Work out the finished part from the listing and answer in its coordinate system (mm). A direction names the side the tool comes from. Give positions to 0.01 mm unless a question says otherwise; leave off trailing zeros. Write each loop counter-clockwise with the first axis right and the second up, starting at its lowest first coordinate (ties: lowest second). Pieces come first, ordered by that corner, then holes. Notation, with made-up numbers: (38, 78) - (64, 78) arc R22 cw to (64, 108) - close; hole circle Ø6 at (-35.75, 40.5). An arc over 180 degrees is marked (long way). Write item = value, one per line.
from build123d import *

# Parameters (mm, degrees)
SKETCH1_W               = 48
SKETCH1_H               = 6
BOSS_EXTRUDE1_DEPTH     = 205
FILLET1_R               = 25
SKETCH2_R               = 2.55
CUT_EXTRUDE1_DEPTH      = 207.487287744
LPATTERN1_COUNT         = 10
LPATTERN1_PITCH         = 10
CUT_EXTRUDE2_DEPTH      = 207.421898063
CUT_EXTRUDE2_DEPTH_BACK = 207.421898063
SKETCH12_W              = 15
SKETCH12_H              = 55
FILLET2_R               = 5


with BuildPart() as part:
    # Sketch1 → Boss-Extrude1 (new body)
    with BuildSketch(Plane(origin=(0, 0, 0), x_dir=(1, 0, 0), z_dir=(0, 1, 0))):
        Rectangle(SKETCH1_W, SKETCH1_H)
    extrude(amount=BOSS_EXTRUDE1_DEPTH)

    # Fillet1
    # the kernel refuses this fillet: 25 mm, written as the material it takes off along each edge
    with BuildSketch(Plane(origin=(-24, 0, 65.5), x_dir=(0, 1, 0), z_dir=(0, 0, -1)), Plane(origin=(24, 0, -65.5), x_dir=(0, 1, 0), z_dir=(0, 0, 1))) as fillet1_piece_1:
        with BuildLine():
            CenterArc((FILLET1_R, FILLET1_R), FILLET1_R, 180, 90)
            Line((0, FILLET1_R), (0, 0))
            Line((0, 0), (FILLET1_R, 0))
        make_face()
    extrude(amount=131, mode=Mode.SUBTRACT)

    # Sketch2 → Cut-Extrude1 (cut, through all)
    with BuildSketch(Plane.XY.offset(3)):
        with Locations((0, 12.5)):
            Circle(SKETCH2_R)
    cut_extrude1 = extrude(amount=-CUT_EXTRUDE1_DEPTH, mode=Mode.SUBTRACT)

    # LPattern1: Cut-Extrude1 ×10
    with Locations(*[(0, i * LPATTERN1_PITCH, 0) for i in range(1, LPATTERN1_COUNT)]):
        add(cut_extrude1, mode=Mode.SUBTRACT)

    # Sketch12 → Cut-Extrude2 (cut, two sides: drawn at the far end of the back side and taken through both)
    with BuildSketch(Plane.XY.offset(-CUT_EXTRUDE2_DEPTH_BACK)):
        with Locations((-16.5, 152.5)):
            Rectangle(SKETCH12_W, SKETCH12_H)
        with Locations((16.5, 152.5)):
            Rectangle(SKETCH12_W, SKETCH12_H)
    extrude(amount=CUT_EXTRUDE2_DEPTH + CUT_EXTRUDE2_DEPTH_BACK, mode=Mode.SUBTRACT)

    # Fillet2
    fillet2_edges = [part.edges().sort_by_distance(p)[0] for p in [
        (-24, 205, 0),
        (24, 205, 0),
        (-24, 125, 0),
        (-24, 180, 0),
        (-9, 180, 0),
        (-9, 125, 0),
        (24, 125, 0),
        (9, 125, 0),
        (9, 180, 0),
        (24, 180, 0),
    ]]
    fillet(fillet2_edges, radius=FILLET2_R)


solid = part.part
1. Given pin 1 (8 mm diameter, centred on x = 0, y = 82.5, fed in from +Z); pin 2 (4 mm diameter, centred on x = 0, y = 92.5, fed in from -Z); pin 3 (3 mm diameter, centred on y = 157.5, z = -1.5, fed in from -X); pin 4 (1.5 mm diameter, centred on x = -17, z = 0, fed in from -Y), each flat-ended and moving along its own axis, determine where each tip first touches the part or whether it passes through.
Solution:
pin_1 = 3
pin_2 = through
pin_3 = -9
pin_4 = 6.9
2. Find section A-A, the plane y = 42.5. Give the vertices of the cut face in (x, z), then the cut area to 3 significant figures.
Solution:
outline = (-24, -3) - (-2.55, -3) - (-2.55, 3) - (-24, 3) - close; (2.55, -3) - (24, -3) - (24, 3) - (2.55, 3) - close
area = 257 mm^2
3. Straight lines are drawn through the part: line 1 (X direction, y = 137, z = -2.6); line 2 (Y direction, x = -10, z = -1.6); line 3 (X direction, y = 82, z = -2.7). For each, find the intervals that lie inside material, in ascending order.
Solution:
line_1 = -9 to 9
line_2 = 2.55 to 127, 178 to 205
line_3 = -24 to -2.5, 2.5 to 24
4. A tool of negligible diameter and unlimited length cuts with its end or side. For faces 4 (the cylindrical face through (1.37, 84.65, 0.04)), 5 (the cylindrical face through (11, 126, 0)), 6 (the cylindrical face through (-23, 182, 0)), from which of +Z, -Z, +X, -X, +Y, -Y can it reach the whole face along a straight path? Write none if from no direction.
Solution:
face_4 = +Z, -Z
face_5 = +Z, -Z, +X
face_6 = +Z, -Z, -X
5. Find section C-C, the plane z = -1.2. Give the number of separate pieces and of enclosed holes in the cut face, then the cut area to 3 significant figures.
Solution:
separate_pieces = 1
enclosed_holes = 10
area = 7,710 mm^2
6. Find section D-D, the plane y = 149. Give the vertices of the cut face in (x, z).
Solution:
outline = (-9, -3) - (9, -3) - (9, 3) - (-9, 3) - close
7. Find section B-B, the plane x = -16. Give the vertices of the cut face in (y, z), then the cut area to 3 significant figures.
Solution:
outline = (6.67, -3) - (125, -3) - (125, 3) - (6.67, 3) - close; (180, -3) - (205, -3) - (205, 3) - (180, 3) - close
area = 860 mm^2
8. For a pull along Y with two mould halves and no side action, classify faces 1 (the cylindrical face through (-0.33, 55.03, 0.04)), 2 (the flat face through (-24, 72, 0)), 3 (the cylindrical face through (16.841, 7.487, -0.042)) as pulls with the +Y half, pulls with the -Y half, needs draft (parallel to the pull), parting line crosses it, or undercut.
Solution:
face_1 = undercut
face_2 = needs draft
face_3 = pulls with the -Y half
